from build123d import *

# Parameters (mm, degrees)
F0_W     = 50.8
F0_H     = 50.8
F1_DEPTH = 876.3
F2_W     = 44.45
F2_H     = 44.45
F3_DEPTH = 876.3
F4_R     = 9.525
F5_R     = 12.7
F6_DEPTH = 50.8
F7_R     = 12.7
F8_DEPTH = 127


with BuildPart() as f1:
    # F0 (on Right) → F1 (new body)
    with BuildSketch(Plane.YZ):
        with Locations((25.4, 25.4)):
            Rectangle(F0_W, F0_H)
    extrude(amount=-F1_DEPTH)

    # F2 (on face) → F3 (cut)
    with BuildSketch(Plane.YZ):
        with Locations((25.4, 25.4)):
            Rectangle(F2_W, F2_H)
    extrude(amount=-F3_DEPTH, mode=Mode.SUBTRACT)

    # F4
    f4_edges = [f1.edges().sort_by_distance(p)[0] for p in [
        (-438.15, 3.175, 3.175),
        (-438.15, 47.625, 3.175),
        (-438.15, 47.625, 47.625),
        (-438.15, 3.175, 47.625),
        (-438.15, 50.8, 0),
        (-438.15, 50.8, 50.8),
        (-438.15, 0, 50.8),
        (-438.15, 0, 0),
    ]]
    fillet(f4_edges, radius=F4_R)

    # F5 (on face) → F6 (cut)
    with BuildSketch(Plane.XY.offset(50.8)):
        with Locations((-844.55, 25.4)):
            Circle(F5_R)
    extrude(amount=-F6_DEPTH, mode=Mode.SUBTRACT)

    # F7 (on face) → F8 (join)
    with BuildSketch(Plane(origin=(0, 0, 0), x_dir=(1, 0, 0), z_dir=(0, 0, -1))):
        with Locations((-844.55, -25.4)):
            Circle(F7_R)
    extrude(amount=-F8_DEPTH)


solid = f1.part
Here's how the part is built. I have some questions about the finished solid (model axes, mm). A direction names the side the tool comes from. Coordinates: 2 decimals unless noted, no trailing zeros. Order: outer loops, then holes, each group sorted by start corner. A loop starts at its lowest first (then second) coordinate and runs counter-clockwise, first axis right, second up. Notation, with made-up numbers: M 29.25,77.25 L 36.25,77.25 A29 ccw 36.25,106.25 Z; hole C -8.5,88 d9. An arc over 180 degrees is marked long. Answer as CSV lines item,"result".
Item 1: On a 3-axis mill with a long thin cutter (end or side, diameter ignored), from which of +Z, -Z, +X, -X, +Y, -Y can I reach the whole of each face in a straight line? I mean faces 5 (the face through (-867, 25, 3.175)), 6 (the face through (-854.628, 33.128, 25.089)), 7 (the face through (-416, 25, 47.625)), 8 (the face through (-432, 3.175, 25)), 9 (the face through (0, 27, 3)). Say none if no direction works.
Results found:
face 5,"-X"
face 6,"none"
face 7,"+X"
face 8,"+X, -X"
face 9,"+Z, -Z, +X, +Y, -Y"
Item 2: We'd pull the mould along Z, two halves only. Please class faces 1 (the face through (-854.628, 33.128, 88.367)), 2 (the face through (-432, 47.625, 25)), 3 (the face through (-432, 25, 0)), 4 (the face through (-432, 25, 50.8)): +Z half, -Z half, draft (parallel to the pull), parting line (faces both ways), or undercut.
Results found:
face 1,"draft"
face 2,"undercut"
face 3,"-Z half"
face 4,"+Z half"
Item 3: Imagine slicing it at A-A on x = -337.5. Write out the boundary of the cut face in (y, z) (3 decimals).
Results found:
outline,"M 0,9.525 A9.525 ccw 9.525,0 L 41.275,0 A9.525 ccw 50.8,9.525 L 50.8,41.275 A9.525 ccw 41.275,50.8 L 9.525,50.8 A9.525 ccw 0,41.275 Z; hole M 3.175,12.7 A9.525 ccw 12.7,3.175 L 38.1,3.175 A9.525 ccw 47.625,12.7 L 47.625,38.1 A9.525 ccw 38.1,47.625 L 12.7,47.625 A9.525 ccw 3.175,38.1 Z"
Item 4: Imagine slicing it at B-B on y = 25.4. Write out the boundary of the cut face in (x, z) (3 decimals), plus the area to 3 significant figures.
Results found:
outline,"M -876.3,0 L 0,0 L 0,3.175 L -831.85,3.175 L -831.85,47.625 L 0,47.625 L 0,50.8 L -831.85,50.8 L -831.85,127 L -857.25,127 L -857.25,50.8 L -876.3,50.8 L -876.3,47.625 L -857.25,47.625 L -857.25,3.175 L -876.3,3.175 Z"
area,"8,630 mm2"
Item 5: For pin 1 (20.5 mm diameter, centred on x = -330.5, y = 22.5, fed in from +Z); pin 2 (1 mm diameter, centred on y = 14.5, z = 75, fed in from +X), each with a flat end and sliding along its axis, tell me the tip position at first contact or that it passes through.
Results found:
pin 1,"z = 50.8"
pin 2,"x = -837.26"
Item 6: Imagine slicing it at C-C on z = 88. Write out the boundary of the cut face in (x, y), plus the area to 3 significant figures.
Results found:
outline,"C -844.55,25.4 d25.4"
area,"507 mm2"
Item 7: If I drill on line 1 (Y direction, x = -273.5, z = 22) (3 decimals); line 2 (Y direction, x = -836, z = 39), over which ranges is the centre line in solid material (lowest first)?
Results found:
line 1,"0 to 3.175, 47.625 to 50.8"
line 2,"0 to 3.22, 16.01 to 34.79, 47.58 to 50.8"
